Design review of the part built by this model. Coordinates are the model's own, in mm. Face numbers are marked on the shaded views. A direction names the side the tool comes from. Round coordinates to 2 decimals unless told otherwise and drop trailing zeros. Order: outer loops, then holes, each group sorted by start corner. A loop starts at its lowest first (then second) coordinate and runs counter-clockwise, first axis right, second up. Notation, with made-up numbers: M -1.5,10.25 L 17.5,10.25 A7 ccw 17.5,18.25 Z; hole C 9.25,42.5 d2. An arc over 180 degrees is marked long. Write each question's results on one line, items separated by ' | '. Start each with the question number.
Item 1: Take a section at B-B, the plane x = 17. Write out the cut boundary in (y, z).
Item 2: Take a section at A-A, the plane z = 0. Write out the cut boundary in (x, y), plus the area to 3 significant figures.
Item 3: Machinability: for the marked faces 5, 6, 7, 8 and 9, which of the approach directions +Z, -Z, +X, -X, +Y, -Y give a long, thin tool a straight path to every point of the face, cutting with its end or side? Answer none if there is none.
Item 4: The part is to be moulded in two halves that separate along Z. For the marked faces 1, 2, 3 and 4, say which applies: +Z half, -Z half, draft (parallel to the pull), parting line (faces both ways), or undercut.
Item 5: Wall thickness on line 1 (Z direction, x = 14, y = 0); line 2 (Z direction, x = -25, y = 0); line 3 (Z direction, x = -9, y = 15.5): over which ranges is each line inside the solid? List them lowest first. Write a range as [from, to].
Item 6: Clearance check with flat-ended pins moving along their axes: pin 1 (6.5 mm diameter, centred on x = 5, y = -12.5, fed in from +Z); pin 2 (5 mm diameter, centred on y = -5, z = -15.5, fed in from -X); pin 3 (16 mm diameter, centred on x = -2, y = 12.5, fed in from +Z); pin 4 (5 mm diameter, centred on y = 0, z = 0, fed in from +X). State where each tip first meets the part, or that it passes through.
Item 7: Take a section at C-C, the plane y = 17. Write out the cut boundary in (x, z).
Item 8: Take a section at D-D, the plane x = -30.5. Write out the cut boundary in (y, z).
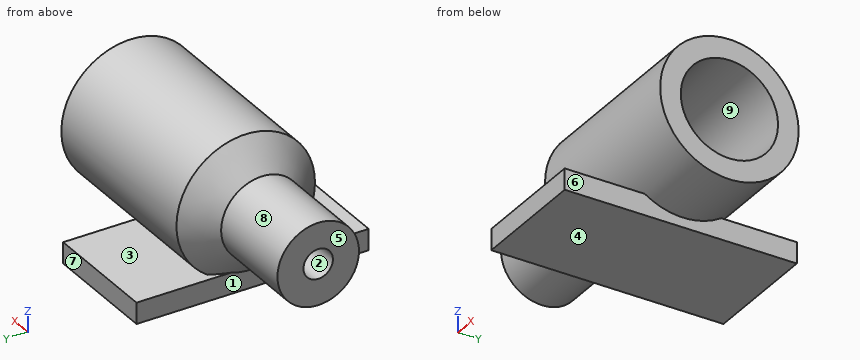
```python
from build123d import *

# Parameters (mm, degrees)
F2_W     = 49.1305962205
F2_H     = 4.4664181769
F3_DEPTH = 12.5


# Not quite as in the source:
# - a feature names something its author has since deleted; it is built from what else it names


with BuildPart() as f1:
    # F0 (on Top) → F1 (revolve)
    with BuildSketch(Plane.XY):
        Polygon((-35.6138087809, 8.6301378906), (-35.6138087809, 3.1164383981), (-16.4602123841, 3.1164383981), (-13.8548975913, 5.887503858), (-10.9075363725, 3.1164383981), (-4.8190304078, 3.1164383981), (-4.8190304078, 10.2874673903), (28.3264927566, 10.2874673903), (28.3264927566, 14.6608594805), (-10.9075363725, 14.6608594805), (-16.4212342352, 8.6301378906), align=None)
    revolve(axis=Axis((-1.5279836953, 0, 0), (1, 0, 0)))

    # F2 (on Right) → F3 (join, symmetric)
    with BuildSketch(Plane.YZ):
        with Locations((-0.4701502621, -14.4570898265)):
            Rectangle(F2_W, F2_H)
    extrude(amount=F3_DEPTH, both=True)


solid = f1.part
```
Results list:
1) outline: C 0,0 d29.32; hole C 0,0 d20.57
2) outline: M -35.61,-8.63 L -16.42,-8.63 L -10.91,-14.66 L 28.33,-14.66 L 28.33,-10.29 L -4.82,-10.29 L -4.82,-3.12 L -10.91,-3.12 L -13.85,-5.89 L -16.46,-3.12 L -35.61,-3.12 Z; M -35.61,3.12 L -16.46,3.12 L -13.85,5.89 L -10.91,3.12 L -4.82,3.12 L -4.82,10.29 L 28.33,10.29 L 28.33,14.66 L -10.91,14.66 L -16.42,8.63 L -35.61,8.63 Z | area: 721 mm²
3) face 5: +Z, -Z, -X, +Y, -Y | face 6: -Z, +X | face 7: +Z, -Z, +X, -X, +Y | face 8: -X | face 9: +X
4) face 1: draft | face 2: undercut | face 3: undercut | face 4: -Z half
5) line 1: [-14.66, -10.29], [10.29, 14.66] | line 2: [-8.63, -3.12], [3.12, 8.63] | line 3: [-16.69, -12.22]
6) pin 1: z = 11.37 | pin 2: x = -12.5 | pin 3: z = 13.95 | pin 4: through
7) outline: M -12.5,-16.69 L 12.5,-16.69 L 12.5,-12.22 L -12.5,-12.22 Z
8) outline: C 0,0 d17.26; hole C 0,0 d6.23
